from build123d import *

# Parameters (mm, degrees)
SKETCH_1_R          = 5.25
EXTRUDE_1_DEPTH     = 15
CUT_EXTRUDE_START   = -10
CUT_EXTRUDE_1_DEPTH = 10
EXTRUDE_2_DEPTH     = 18
SKETCH_4_R          = 1.5
CUT_EXTRUDE_2_DEPTH = 39.304699451


with BuildPart() as part:
    # 草图1 → 凸台-拉伸1 (new body)
    with BuildSketch(Plane.XY):
        with BuildLine():
            Line((-11.489125293, -8), (11.489125293, -8))
            ThreePointArc((11.489125293, -8), (0, 14), (-11.489125293, -8))
        make_face()
        Circle(SKETCH_1_R, mode=Mode.SUBTRACT)
    extrude(amount=EXTRUDE_1_DEPTH)

    # 草图2 → 切除-拉伸1 (cut)
    with BuildSketch(Plane.XY.offset(15).offset(CUT_EXTRUDE_START)):
        with BuildLine():
            Line((-13.416407865, 4), (13.416407865, 4))
            ThreePointArc((13.416407865, 4), (0, 14), (-13.416407865, 4))
        make_face()
    extrude(amount=CUT_EXTRUDE_1_DEPTH, mode=Mode.SUBTRACT)

    # 草图3 → 凸台-拉伸2 (add)
    with BuildSketch(Plane.XY.offset(15)):
        with BuildLine():
            Line((-7.123903424, 5.5), (7.123903424, 5.5))
            ThreePointArc((7.123903424, 5.5), (9, 0), (7.123903424, -5.5))
            Line((7.123903424, -5.5), (-7.123903424, -5.5))
            ThreePointArc((-7.123903424, -5.5), (-9, 0), (-7.123903424, 5.5))
        make_face()
    extrude(amount=EXTRUDE_2_DEPTH)

    # 草图4 → 切除-拉伸2 (cut, through all)
    with BuildSketch(Plane(origin=(0, 5.5, 0), x_dir=(1, 0, 0), z_dir=(0, 1, 0))):
        with Locations(Location((4.5, -26.46, 0), (0, 0, 270))):
            Circle(SKETCH_4_R)
        with Locations(Location((-4.5, -26.46, 0), (0, 0, 180))):
            Circle(SKETCH_4_R)
    extrude(amount=-CUT_EXTRUDE_2_DEPTH, mode=Mode.SUBTRACT)


solid = part.part
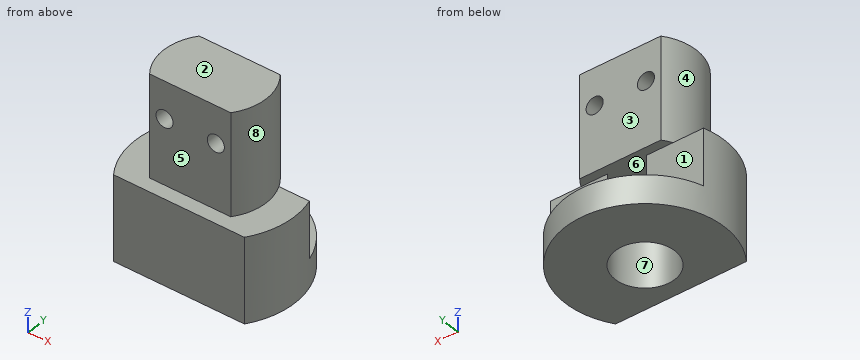
The model under review builds one solid part; all positions refer to its coordinate system, in mm. Face numbers are marked on the shaded views. A direction names the side the tool comes from. Give positions to 0.01 mm unless a question says otherwise; leave off trailing zeros. Order: outer loops, then holes, each group sorted by start corner. A loop starts at its lowest first (then second) coordinate and runs counter-clockwise, first axis right, second up. Notation, with made-up numbers: (66, -30) -> (77, -30) arc R22 cw to (77, 7) -> close; hole circle Ø6 at (2.5, 45). An arc over 180 degrees is marked (long way). Write item = value, one per line. Start each with the question number.
(1) Draft analysis for pull direction Z (two halves, no side actions). For the marked faces 1, 2 and 3, state which applies: +Z half, -Z half, draft (parallel to the pull), parting line (faces both ways), or undercut.
(2) For L1, parallel to X at y = 0, z = 11; L2, parallel to X at y = -1.5, z = 27.5; L3, parallel to Z at x = -8, y = -6, list the stretches that pass through material, from the lowest coordinate up. Write a range as from..to.
(3) Tool access review of the marked faces 4, 5, 6, 7 and 8: name each direction out of +Z, -Z, +X, -X, +Y, -Y from which nothing blocks a thin tool from reaching the whole face with its end or side.
(4) Take a section at C-C (x = -4.5). Write out the cut boundary in (y, z), plus the area to 3 significant figures.
(5) Take a section at D-D (z = 8.5). Write out the cut boundary in (x, y).
(6) Take a section at A-A (y = 0). Write out the cut boundary in (x, z).
(7) Take a section at B-B (z = 26.46). Write out the cut boundary in (x, y), plus the area to 3 significant figures.
(8) For pin 1 Ø15.5 at (x, z) = (-2.5, 24) entering from -Y; pin 2 Ø3 at (x, z) = (-8.5, 10) entering from +Y; pin 3 Ø6.5 at (x, y) = (0, 0) entering from -Z, all flat-tipped, find the tip position at first contact; note any pin that passes through.
Returned:
q1.face_1 = undercut
q1.face_2 = +Z half
q1.face_3 = draft
q2.L1 = -14..-5.25, 5.25..14
q2.L2 = -8.87..-5.58, -3.42..3.42, 5.58..8.87
q2.L3 = 0..15
q3.face_4 = +Z, -X
q3.face_5 = +Z, +X, -X, -Y
q3.face_6 = none
q3.face_7 = -Z
q3.face_8 = +Z, +X
q4.outline = (-8, 0) -> (-2.7, 0) -> (-2.7, 15) -> (2.7, 15) -> (2.7, 0) -> (13.26, 0) -> (13.26, 5) -> (4, 5) -> (4, 15) -> (5.5, 15) -> (5.5, 24.96) -> (-5.5, 24.96) -> (-5.5, 15) -> (-8, 15) -> close; (-5.5, 27.96) -> (5.5, 27.96) -> (5.5, 33) -> (-5.5, 33) -> close
q4.area = 310 mm²
q5.outline = (-13.42, 4) arc R14 ccw to (-11.49, -8) -> (11.49, -8) arc R14 ccw to (13.42, 4) -> (3.4, 4) arc R5.25 cw (long way) to (-3.4, 4) -> close
q6.outline = (-14, 0) -> (-5.25, 0) -> (-5.25, 15) -> (5.25, 15) -> (5.25, 0) -> (14, 0) -> (14, 15) -> (9, 15) -> (9, 33) -> (-9, 33) -> (-9, 15) -> (-14, 15) -> close; hole circle Ø3 at (-4.5, 26.46); hole circle Ø3 at (4.5, 26.46)
q7.outline = (-7.12, -5.5) -> (-6, -5.5) -> (-6, 5.5) -> (-7.12, 5.5) arc R9 ccw to start; (-3, -5.5) -> (3, -5.5) -> (3, 5.5) -> (-3, 5.5) -> close; (6, -5.5) -> (7.12, -5.5) arc R9 ccw to (7.12, 5.5) -> (6, 5.5) -> close
q7.area = 119 mm²
q8.pin_1 = -5.5
q8.pin_2 = 4
q8.pin_3 = 15
